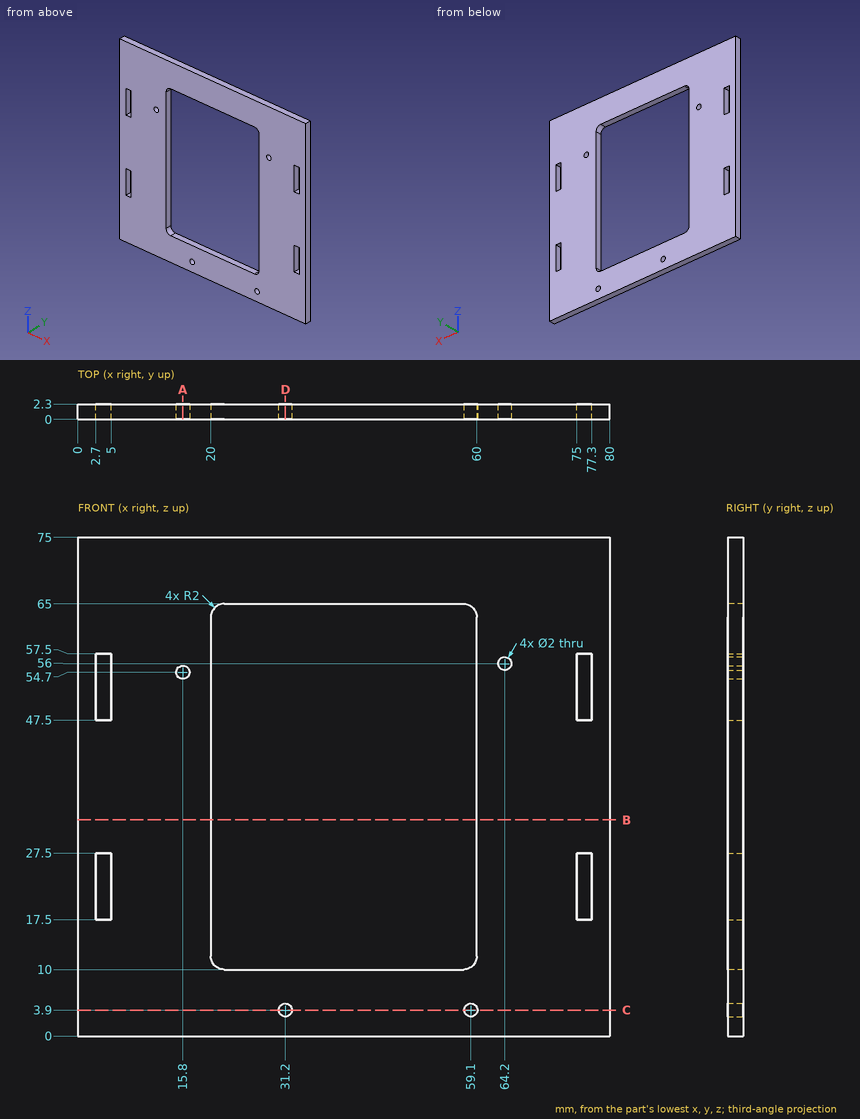
For this review, use the dimensioned drawing (mm, ordinates from the lowest corner) and the shaded views. Give positions to 0.01 mm unless a question says otherwise; leave off trailing zeros. Order: outer loops, then holes, each group sorted by start corner. A loop starts at its lowest first (then second) coordinate and runs counter-clockwise, first axis right, second up. Notation, with made-up numbers: (-16.75, 86) - (8.25, 86) arc R17 ccw to (8.25, 92) - close; hole circle Ø4 at (76.5, 68.5). An arc over 180 degrees is marked (long way). Write item = value, one per line. Start each with the question number.
Q1. To check wall thickness, follow L1, parallel to X at y = 0.95, z = 27; L2, parallel to Z at x = 31.2, y = 0.8; L3, parallel to X at y = 1.1, z = 34. State the ranges of each line that lie inside material, in increasing order. Write a range as from..to.
Q2. We need section B-B on z = 32.5. State the section outline as (x, y) points, plus the area to 3 significant figures.
Q3. We need section D-D on x = 31.2. State the section outline as (y, z) points.
Q4. We need section A-A on x = 15.8. State the section outline as (y, z) points.
Q5. We need section C-C on z = 3.9. State the section outline as (x, y) points, plus the area to 3 significant figures.
Working result:
q1.L1 = 0..2.7, 5..20, 60..75, 77.3..80
q1.L2 = 0..2.9, 4.9..10, 65..75
q1.L3 = 0..20, 60..80
q2.outline = (0, 0) - (20, 0) - (20, 2.3) - (0, 2.3) - close; (60, 0) - (80, 0) - (80, 2.3) - (60, 2.3) - close
q2.area = 92.0 mm²
q3.outline = (0, 0) - (2.3, 0) - (2.3, 2.9) - (0, 2.9) - close; (0, 4.9) - (2.3, 4.9) - (2.3, 10) - (0, 10) - close; (0, 65) - (2.3, 65) - (2.3, 75) - (0, 75) - close
q4.outline = (0, 0) - (2.3, 0) - (2.3, 53.7) - (0, 53.7) - close; (0, 55.7) - (2.3, 55.7) - (2.3, 75) - (0, 75) - close
q5.outline = (0, 0) - (30.2, 0) - (30.2, 2.3) - (0, 2.3) - close; (32.2, 0) - (58.1, 0) - (58.1, 2.3) - (32.2, 2.3) - close; (60.1, 0) - (80, 0) - (80, 2.3) - (60.1, 2.3) - close
q5.area = 175 mm²
